from build123d import *

# Parameters (mm, degrees)
SKETCH1_W           = 5.8
SKETCH1_H           = 5
BOSS_EXTRUDE1_DEPTH = 0.8
SKETCH2_W           = 4.9
SKETCH2_H           = 2.9
BOSS_EXTRUDE2_DEPTH = 1.8
FILLET1_R           = 0.6
BOSS_EXTRUDE3_DEPTH = 2.34


with BuildPart() as part:
    # Sketch1 → Boss-Extrude1 (new body)
    with BuildSketch(Plane.XZ):
        with Locations((2.9, 112.5)):
            Rectangle(SKETCH1_W, SKETCH1_H)
    extrude(amount=-BOSS_EXTRUDE1_DEPTH)

    # Sketch2 → Boss-Extrude2 (add)
    with BuildSketch(Plane(origin=(0, 0.8, 0), x_dir=(-1, 0, 0), z_dir=(0, 1, 0))):
        with Locations((-3.35, 112.5)):
            Rectangle(SKETCH2_W, SKETCH2_H)
    extrude(amount=BOSS_EXTRUDE2_DEPTH)

    # Fillet1
    fillet1_edges = [part.edges().sort_by_distance(p)[0] for p in [
        (5.8, 1.7, 113.95),
        (5.8, 1.7, 111.05),
        (0.9, 1.7, 111.05),
        (0.9, 1.7, 113.95),
        (0, 0.4, 115),
        (5.8, 0.4, 115),
        (5.8, 0.4, 110),
        (0, 0.4, 110),
    ]]
    fillet(fillet1_edges, radius=FILLET1_R)

    # Sketch3 → Boss-Extrude3 (add)
    with BuildSketch(Plane.XZ):
        with BuildLine():
            Line((0.6, 110), (5.2, 110))
            ThreePointArc((5.2, 110), (5.624264069, 110.175735931), (5.8, 110.6))
            Line((5.8, 110.6), (5.8, 114.4))
            ThreePointArc((5.8, 114.4), (5.624264069, 114.824264069), (5.2, 115))
            Line((5.2, 115), (0.6, 115))
            ThreePointArc((0.6, 115), (0.175735931, 114.824264069), (0, 114.4))
            Line((0, 114.4), (0, 110.6))
            ThreePointArc((0, 110.6), (0.175735931, 110.175735931), (0.6, 110))
        make_face()
    extrude(amount=BOSS_EXTRUDE3_DEPTH)


solid = part.part
Geometry check sheet. Reference: the model listing, model coordinates, mm. A direction names the side the tool comes from. Give positions to 0.01 mm unless a question says otherwise; leave off trailing zeros. Loops run counter-clockwise (first coordinate to the right, second up) from the corner with the lowest first, then second, coordinate; pieces in that order, holes last.
(1) Depth check by flat-ended pin: pin 1 Ø0.9 at (x, y) = (4, 1.5) entering from -Z; pin 2 Ø0.5 at (y, z) = (1.5, 112) entering from -X. Enter the tip coordinate at first touch or a pass-through.
From the geometry:
pin 1: stops at z = 111.05
pin 2: stops at x = 0.9
(2) Section check A-A on x = 1.65. Record the cut outline in (y, z).
From the geometry:
outline: (-2.34, 110) - (0.8, 110) - (0.8, 111.05) - (2.6, 111.05) - (2.6, 113.95) - (0.8, 113.95) - (0.8, 115) - (-2.34, 115) - close
(3) Section check D-D on z = 110.35. Record the cut outline in (x, y), then the cut area to 3 significant figures.
From the geometry:
outline: (0.05, -2.34) - (5.75, -2.34) - (5.75, 0.8) - (0.05, 0.8) - close
area: 17.9 mm2
(4) Section check C-C on z = 111.95. Record the cut outline in (x, y), then the cut area to 3 significant figures.
From the geometry:
outline: (0, -2.34) - (5.8, -2.34) - (5.8, 2.6) - (0.9, 2.6) - (0.9, 0.8) - (0, 0.8) - close
area: 27.0 mm2
(5) Section check B-B on y = 2. Record the cut outline in (x, z).
From the geometry:
outline: (0.9, 111.65) arc R0.6 ccw to (1.5, 111.05) - (5.2, 111.05) arc R0.6 ccw to (5.8, 111.65) - (5.8, 113.35) arc R0.6 ccw to (5.2, 113.95) - (1.5, 113.95) arc R0.6 ccw to (0.9, 113.35) - close
(6) Set-up check for faces 1 (the flat face through (3, 2, 111.05)), 2 (the flat face through (3, 2, 113.95)), 3 (the flat face through (5.8, 0, 112)), 4 (the flat face through (0.9, 2, 112)), 5 (the flat face through (3, -2.34, 113)): record each of +Z, -Z, +X, -X, +Y, -Y from which the full face is reachable in a straight line by a thin tool's end or side.
From the geometry:
face 1: -Z, +X, -X, +Y
face 2: +Z, +X, -X, +Y
face 3: +Z, -Z, +X, +Y, -Y
face 4: +Z, -Z, -X, +Y
face 5: +Z, -Z, +X, -X, -Y
(7) Thickness scan on L1, parallel to Y at x = 0.5, z = 112.95; L2, parallel to Z at x = 4.25, y = 1.4. Record the ranges inside material, lowest first.
From the geometry:
L1: y = -2.34 to 0.8
L2: z = 111.05 to 113.95
